Here's how the part is built. I have some questions about the finished solid (model axes, mm). A direction names the side the tool comes from. Round coordinates to 2 decimals unless told otherwise and drop trailing zeros. Order: outer loops, then holes, each group sorted by start corner. A loop starts at its lowest first (then second) coordinate and runs counter-clockwise, first axis right, second up.
```python
from build123d import *

# Parameters (mm, degrees)
SKETCH6_R           = 24
SKETCH6_R_2         = 1.55
SKETCH6_R_3         = 8.5
BOSS_EXTRUDE1_DEPTH = 17
SKETCH8_R           = 3.5
CUT_EXTRUDE6_DEPTH  = 3
SKETCH9_R           = 18
CUT_EXTRUDE7_DEPTH  = 13


with BuildPart() as part:
    # Sketch6 → Boss-Extrude1 (new body)
    with BuildSketch(Plane.XY):
        Circle(SKETCH6_R)
        with Locations((0, 20)):
            Circle(SKETCH6_R_2, mode=Mode.SUBTRACT)
        with Locations((14.142135624, 14.142135624)):
            Circle(SKETCH6_R_2, mode=Mode.SUBTRACT)
        with Locations((20, 0)):
            Circle(SKETCH6_R_2, mode=Mode.SUBTRACT)
        with Locations((14.142135624, -14.142135624)):
            Circle(SKETCH6_R_2, mode=Mode.SUBTRACT)
        with Locations((0, -20)):
            Circle(SKETCH6_R_2, mode=Mode.SUBTRACT)
        with Locations((-14.142135624, -14.142135624)):
            Circle(SKETCH6_R_2, mode=Mode.SUBTRACT)
        with Locations((-20, 0)):
            Circle(SKETCH6_R_2, mode=Mode.SUBTRACT)
        with Locations((-14.142135624, 14.142135624)):
            Circle(SKETCH6_R_2, mode=Mode.SUBTRACT)
        Circle(SKETCH6_R_3, mode=Mode.SUBTRACT)
    extrude(amount=BOSS_EXTRUDE1_DEPTH)

    # Sketch8 → Cut-Extrude6 (cut)
    with BuildSketch(Plane(origin=(0, 0, 0), x_dir=(-1, 0, 0), z_dir=(0, 0, -1))):
        with Locations((0, 20)):
            Circle(SKETCH8_R)
        with Locations((14.142135624, 14.142135624)):
            Circle(SKETCH8_R)
        with Locations((20, 0)):
            Circle(SKETCH8_R)
        with Locations((14.142135624, -14.142135624)):
            Circle(SKETCH8_R)
        with Locations((0, -20)):
            Circle(SKETCH8_R)
        with Locations((-14.142135624, -14.142135624)):
            Circle(SKETCH8_R)
        with Locations((-20, 0)):
            Circle(SKETCH8_R)
        with Locations((-14.142135624, 14.142135624)):
            Circle(SKETCH8_R)
    extrude(amount=-CUT_EXTRUDE6_DEPTH, mode=Mode.SUBTRACT)

    # Sketch9 → Cut-Extrude7 (cut)
    with BuildSketch(Plane.XY.offset(17)):
        Circle(SKETCH9_R)
    extrude(amount=-CUT_EXTRUDE7_DEPTH, mode=Mode.SUBTRACT)


solid = part.part
```
1. If we section it at C-C, the plane y = -20: Write out the boundary of the cut face in (x, z), and give its area (3 significant figures).
Evaluation:
outline: (-13.27, 0) - (-3.5, 0) - (-3.5, 3) - (-1.55, 3) - (-1.55, 17) - (-13.27, 17) - close; (1.55, 3) - (3.5, 3) - (3.5, 0) - (13.27, 0) - (13.27, 17) - (1.55, 17) - close
area: 387 mm2
2. If we mould it in two halves opening along Y, with no side actions, what happens to faces 1 (the cylindrical face through (12.53, -17.25, 1.48)), 2 (the cylindrical face through (-23.977, 1.055, 8.381)), 3 (the flat face through (10, 0, 0))? For each: released by +Y, released by -Y, zero draft, split by the parting line, or undercut.
Evaluation:
face 1: undercut
face 2: split by the parting line
face 3: zero draft
3. On a 3-axis mill with a long thin cutter (end or side, diameter ignored), from which of +Z, -Z, +X, -X, +Y, -Y can I reach the whole of each face in a straight line? I mean faces 4 (the cylindrical face through (14.98, -12.84, 9.9)), 5 (the cylindrical face through (-2.343, 17.847, 10.591)), 6 (the flat face through (-2, 19, 3)). Say none if no direction works.
Evaluation:
face 4: +Z, -Z
face 5: +Z
face 6: -Z
4. I need wall thicknesses on probe 1 along Y at (x, z) = (0, 12); probe 2 along Y at (x, z) = (2.5, 1); probe 3 along X at (y, z) = (17, 0.5). Which ranges of each line are inside material? Lowest first, please.
Evaluation:
probe 1: y = -24 to -21.55, -18.45 to -18, 18 to 18.45, 21.55 to 24
probe 2: y = -23.87 to -22.45, -17.55 to -8.12, 8.12 to 17.55, 22.45 to 23.87
probe 3: x = -16.94 to -16.16, -12.12 to -1.8, 1.8 to 12.12, 16.16 to 16.94
5. If we section it at A-A, the plane y = 0: Write out the boundary of the cut face in (x, z).
Evaluation:
outline: (-24, 0) - (-23.5, 0) - (-23.5, 3) - (-21.55, 3) - (-21.55, 17) - (-24, 17) - close; (-18.45, 3) - (-16.5, 3) - (-16.5, 0) - (-8.5, 0) - (-8.5, 4) - (-18, 4) - (-18, 17) - (-18.45, 17) - close; (8.5, 0) - (16.5, 0) - (16.5, 3) - (18.45, 3) - (18.45, 17) - (18, 17) - (18, 4) - (8.5, 4) - close; (21.55, 3) - (23.5, 3) - (23.5, 0) - (24, 0) - (24, 17) - (21.55, 17) - close
6. If we section it at D-D, the plane x = 15: Write out the boundary of the cut face in (y, z) (3 decimals).
Evaluation:
outline: (-18.735, 0) - (-17.535, 0) - (-17.535, 3) - (-15.433, 3) - (-15.433, 17) - (-18.735, 17) - close; (-12.851, 3) - (-10.749, 3) - (-10.749, 0) - (10.749, 0) - (10.749, 3) - (12.851, 3) - (12.851, 17) - (9.95, 17) - (9.95, 4) - (-9.95, 4) - (-9.95, 17) - (-12.851, 17) - close; (15.433, 3) - (17.535, 3) - (17.535, 0) - (18.735, 0) - (18.735, 17) - (15.433, 17) - close
7. I'm going to push flat-ended pins straight in: P1, Ø4, axis at x = -14.5, z = 2.5, coming from the +Y side; P2, Ø8, axis at x = 10.5, z = 3.5, coming from the +Y side; P3, Ø4, axis at x = 5, z = 12.5, coming from the +Y side; P4, Ø3, axis at x = 0, y = 20, coming from the -Z side. Where does each tip first touch, or does it pass through?
Evaluation:
P1: stops at y = 20.49
P2: stops at y = 23.1
P3: stops at y = 23.81
P4: passes through
